The model under review builds one solid part; all positions refer to its coordinate system, in mm. A direction names the side the tool comes from. Round coordinates to 2 decimals unless told otherwise and drop trailing zeros. Order: outer loops, then holes, each group sorted by start corner. A loop starts at its lowest first (then second) coordinate and runs counter-clockwise, first axis right, second up.
1) Clearance check with flat-ended pins moving along their axes: P1, Ø12, axis at x = -62, z = -60.5, coming from the +Y side; P2, Ø1.9, axis at x = -40.5, y = 24, coming from the +Z side; P3, Ø8, axis at y = 27, z = -33.5, coming from the -X side. State where each tip first meets the part, or that it passes through.
2) Consider section A-A (z = -1.5). Give the boundary of the cut face in (x, y), then the cut area to 3 significant figures.
3) Mouldability with a two-part tool opening along Z and no side actions: class faces 4 (the face through (-36, 28, -57)), 5 (the face through (-76.47, 10.32, -66.18)), 6 (the face through (-12.7, 23, -3)), 7 (the face through (-90.006, 15, -16)) as pulls with the +Z half, pulls with the -Z half, needs draft (parallel to the pull), parting line crosses it, or undercut.
4) Consider section B-B (y = 8.5). Give the boundary of the cut face in (x, z).
5) Consider section D-D (z = 15.5). Give the boundary of the cut face in (x, y) (3 decimals), then the cut area to 3 significant figures.
6) Machinability: for faces 1 (the face through (-31, 12.7, -68)), 2 (the face through (-38.933, 28.077, 19.139)), 3 (the face through (-79.007, 25.578, -42.599)), which of the approach directions +Z, -Z, +X, -X, +Y, -Y give a long, thin tool a straight path to every point of the face, cutting with its end or side? Answer none if there is none.
7) Consider section C-C (y = 18). Give the boundary of the cut face in (x, z).
8) To check wall thickness, follow L1, parallel to Z at x = -15, y = 25; L2, parallel to Y at x = -14.45, z = 0 (3 decimals); L3, parallel to Z at x = -81, y = 24. State the ranges of each line that lie inside material, in increasing order.
from build123d import *

# Parameters (mm, degrees)
SALIENTE_EXTRUIR1_DEPTH = 38.1
CROQUIS2_W              = 25.4
CROQUIS2_H              = 25.4
CORTAR_EXTRUIR1_DEPTH   = 25.4
CROQUIS3_W              = 64.605839452
CROQUIS3_H              = 25.4
CORTAR_EXTRUIR2_DEPTH   = 25.4
CROQUIS4_W              = 25.4
CROQUIS4_H              = 53.34
CORTAR_EXTRUIR3_DEPTH   = 25.4
CORTAR_EXTRUIR4_DEPTH   = 25.4
CORTAR_EXTRUIR5_DEPTH   = 25.4
CROQUIS7_R              = 3.175
CORTAR_EXTRUIR6_DEPTH   = 50.8
CROQUIS8_R              = 3.175
CORTAR_EXTRUIR7_DEPTH   = 50.8
CROQUIS10_R             = 3.175
CORTAR_EXTRUIR9_DEPTH   = 43.18
CROQUIS11_R             = 3.175
CORTAR_EXTRUIR10_DEPTH  = 50.8
SKETCH1_R               = 6.35
CUT_EXTRUDE1_DEPTH      = 39.1


with BuildPart() as part:
    # Croquis1 → Saliente-Extruir1 (new body)
    with BuildSketch(Plane(origin=(0, 0, 0), x_dir=(1, 0, 0), z_dir=(0, 1, 0))):
        Polygon((25.4, 78.74), (25.4, -12.7), (12.7, -25.4), (-90.005839452, -25.4), (-90.005839452, 58.42), (-54.552420926, 78.74), align=None)
    extrude(amount=SALIENTE_EXTRUIR1_DEPTH)

    # Croquis2 → Cortar-Extruir1 (cut)
    with BuildSketch(Plane(origin=(0, 38.1, 0), x_dir=(1, 0, 0), z_dir=(0, 1, 0))):
        Rectangle(CROQUIS2_W, CROQUIS2_H)
    extrude(amount=-CORTAR_EXTRUIR1_DEPTH, mode=Mode.SUBTRACT)

    # Croquis3 → Cortar-Extruir2 (cut)
    with BuildSketch(Plane(origin=(0, 38.1, 0), x_dir=(1, 0, 0), z_dir=(0, 1, 0))):
        with Locations((-57.702919726, 0)):
            Rectangle(CROQUIS3_W, CROQUIS3_H)
    extrude(amount=-CORTAR_EXTRUIR2_DEPTH, mode=Mode.SUBTRACT)

    # Croquis4 → Cortar-Extruir3 (cut)
    with BuildSketch(Plane(origin=(0, 38.1, 0), x_dir=(1, 0, 0), z_dir=(0, 1, 0))):
        with Locations((0, 52.07)):
            Rectangle(CROQUIS4_W, CROQUIS4_H)
    extrude(amount=-CORTAR_EXTRUIR3_DEPTH, mode=Mode.SUBTRACT)

    # Croquis5 → Cortar-Extruir4 (cut)
    with BuildSketch(Plane(origin=(0, 38.1, 0), x_dir=(1, 0, 0), z_dir=(0, 1, 0))):
        Polygon((-59.011096598, 32.102249098), (-36.601753481, 44.059729647), (-54.977056362, 78.496621719), (-77.024213035, 65.860372741), align=None)
    extrude(amount=-CORTAR_EXTRUIR4_DEPTH, mode=Mode.SUBTRACT)

    # Croquis6 → Cortar-Extruir5 (cut)
    with BuildSketch(Plane(origin=(0, 38.1, 0), x_dir=(1, 0, 0), z_dir=(0, 1, 0))):
        Polygon((-25.397081923, 50.038469922), (-40.712032739, 78.74), (-25.397081923, 78.74), align=None)
        Polygon((-70.215768156, 26.123508824), (-88.047791372, 59.542248253), (-90.005839452, 58.42), (-90.005839452, 26.123508824), align=None)
    extrude(amount=-CORTAR_EXTRUIR5_DEPTH, mode=Mode.SUBTRACT)

    # Croquis7 → Cortar-Extruir6 (cut)
    with BuildSketch(Plane.XY.offset(25.4)):
        with Locations((-40.64, 25.4)):
            Circle(CROQUIS7_R)
    extrude(amount=-CORTAR_EXTRUIR6_DEPTH, mode=Mode.SUBTRACT)

    # Croquis8 → Cortar-Extruir7 (cut)
    with BuildSketch(Plane(origin=(25.4, 0, 0), x_dir=(0, 0, -1), z_dir=(1, 0, 0))):
        with Locations((40.64, 25.4)):
            Circle(CROQUIS8_R)
    extrude(amount=-CORTAR_EXTRUIR7_DEPTH, mode=Mode.SUBTRACT)

    # Croquis10 → Cortar-Extruir9 (cut)
    with BuildSketch(Plane(origin=(25.4, 0, 0), x_dir=(0, 0, -1), z_dir=(1, 0, 0))):
        with Locations((0, 25.4)):
            Circle(CROQUIS10_R)
    extrude(amount=-CORTAR_EXTRUIR9_DEPTH, mode=Mode.SUBTRACT)

    # Croquis11 → Cortar-Extruir10 (cut)
    with BuildSketch(Plane(origin=(-43.804364121, 0, 23.373725379), x_dir=(0.470766951, 0, 0.882257603), z_dir=(-0.882257603, 0, 0.470766951))):
        with Locations((-69.056927347, 25.4)):
            Circle(CROQUIS11_R)
    extrude(amount=-CORTAR_EXTRUIR10_DEPTH, mode=Mode.SUBTRACT)

    # Sketch1 → Cut-Extrude1 (cut, through all)
    with BuildSketch(Plane(origin=(0, 38.1, 0), x_dir=(1, 0, 0), z_dir=(0, 1, 0))):
        with Locations((-30.48, 30.48)):
            Circle(SKETCH1_R)
    extrude(amount=-CUT_EXTRUDE1_DEPTH, mode=Mode.SUBTRACT)


solid = part.part
Answer below:
1. P1: stops at y = 12.7
1. P2: stops at z = -25.4
1. P3: stops at x = -76.12
2. outline: (-90.01, 0) - (25.4, 0) - (25.4, 22.6) - (12.7, 22.6) - (12.7, 12.7) - (-12.7, 12.7) - (-12.7, 22.6) - (-17.78, 22.6) - (-17.78, 28.2) - (-12.7, 28.2) - (-12.7, 38.1) - (-25.4, 38.1) - (-25.4, 12.7) - (-90.01, 12.7) - close; (12.7, 28.2) - (25.4, 28.2) - (25.4, 38.1) - (12.7, 38.1) - close
2. area: 2,010 mm2
3. face 4: undercut
3. face 5: pulls with the -Z half
3. face 6: undercut
3. face 7: needs draft
4. outline: (-90.01, -58.42) - (-54.55, -78.74) - (25.4, -78.74) - (25.4, 12.7) - (12.7, 25.4) - (-90.01, 25.4) - close; hole circle Ø12.7 at (-30.48, -30.48)
5. outline: (-90.006, 0) - (22.6, 0) - (22.6, 38.1) - (-90.006, 38.1) - close; hole circle Ø6.35 at (-40.64, 25.4)
5. area: 4,260 mm2
6. face 1: -Z, +Y
6. face 2: +Z
6. face 3: -X, +Y
7. outline: (-90.01, -26.12) - (-70.22, -26.12) - (-88.05, -59.54) - (-77.02, -65.86) - (-59.01, -32.1) - (-36.6, -44.06) - (-54.98, -78.5) - (-54.55, -78.74) - (-40.71, -78.74) - (-25.4, -50.04) - (-25.4, -78.74) - (-12.7, -78.74) - (-12.7, -25.4) - (12.7, -25.4) - (12.7, -78.74) - (25.4, -78.74) - (25.4, 12.7) - (12.7, 25.4) - (-90.01, 25.4) - (-90.01, 12.7) - (-25.4, 12.7) - (-25.4, -12.7) - (-90.01, -12.7) - close; hole circle Ø12.7 at (-30.48, -30.48); hole (-12.7, -12.7) - (12.7, -12.7) - (12.7, 12.7) - (-12.7, 12.7) - close
8. L1: z = -78.74 to -43.79, -37.49 to -3.15, 3.15 to 25.4
8. L2: y = 0 to 22.225, 28.575 to 38.1
8. L3: z = -63.58 to -46.33, -26.12 to -12.7, 12.7 to 25.4
